```python
from build123d import *

# Parameters (mm, degrees)
F0_W     = 5.588
F0_H     = 23.114
F1_DEPTH = 1.651
F2_W     = 5.75
F2_H     = 23.114
F3_DEPTH = 13.5
F4_R     = 2.1
F5_DEPTH = 25.4
F6_R     = 4
F7_DEPTH = 2.5


with BuildPart() as f1:
    # F0 (on Top) → F1 (new body)
    with BuildSketch(Plane.XY):
        Rectangle(F0_W, F0_H)
    extrude(amount=F1_DEPTH)

    # F2 (on face) → F3 (join)
    with BuildSketch(Plane.XY.offset(1.651)):
        with Locations((3.831, 0)):
            Rectangle(F2_W, F2_H)
    extrude(amount=F3_DEPTH)

    # F4 (on face) → F5 (cut)
    with BuildSketch(Plane.YZ.offset(6.706)):
        with Locations((0, 10.151)):
            Circle(F4_R)
    extrude(amount=-F5_DEPTH, mode=Mode.SUBTRACT)

    # F6 (on face) → F7 (cut)
    with BuildSketch(Plane(origin=(0.956, 0, 0), x_dir=(0, -1, 0), z_dir=(-1, 0, 0))):
        with Locations((0, 10.151)):
            Circle(F6_R)
    extrude(amount=-F7_DEPTH, mode=Mode.SUBTRACT)


solid = f1.part
```
Design review of the part built by this model. Coordinates are the model's own, in mm. A direction names the side the tool comes from. Round coordinates to 2 decimals unless told otherwise and drop trailing zeros. Write each loop counter-clockwise with the first axis right and the second up, starting at its lowest first coordinate (ties: lowest second). Pieces come first, ordered by that corner, then holes. Notation, with made-up numbers: (45.25, -0.75) -> (97.25, -0.75) arc R34 cw to (97.25, 30.25) -> close; hole circle Ø1 at (88.25, 26). An arc over 180 degrees is marked (long way). Answer in a Markdown table with one row per item.
Q1. Take a section at C-C, the plane z = 6.5. State the section outline as (x, y) points, then the cut area to 3 significant figures.
The answers:
| item | result |
|---|---|
| outline | (0.96, -11.56) -> (6.71, -11.56) -> (6.71, 11.56) -> (0.96, 11.56) -> (0.96, 1.63) -> (3.46, 1.63) -> (3.46, -1.63) -> (0.96, -1.63) -> close |
| area | 125 mm² |
Q2. Take a section at B-B, the plane y = -7. State the section outline as (x, z) points, then the cut area to 3 significant figures.
The answers:
| item | result |
|---|---|
| outline | (-2.79, 0) -> (2.79, 0) -> (2.79, 1.65) -> (6.71, 1.65) -> (6.71, 15.15) -> (0.96, 15.15) -> (0.96, 1.65) -> (-2.79, 1.65) -> close |
| area | 86.9 mm² |
Q3. Take a section at D-D, the plane x = 1.75. State the section outline as (y, z) points, then the cut area to 3 significant figures.
The answers:
| item | result |
|---|---|
| outline | (-11.56, 0) -> (11.56, 0) -> (11.56, 15.15) -> (-11.56, 15.15) -> close; hole circle Ø8 at (0, 10.15) |
| area | 300 mm² |
Q4. Take a section at A-A, the plane y = 0. State the section outline as (x, z) points, then the cut area to 3 significant figures.
The answers:
| item | result |
|---|---|
| outline | (-2.79, 0) -> (2.79, 0) -> (2.79, 1.65) -> (6.71, 1.65) -> (6.71, 8.05) -> (3.46, 8.05) -> (3.46, 6.15) -> (0.96, 6.15) -> (0.96, 1.65) -> (-2.79, 1.65) -> close; (0.96, 14.15) -> (3.46, 14.15) -> (3.46, 12.25) -> (6.71, 12.25) -> (6.71, 15.15) -> (0.96, 15.15) -> close |
| area | 53.2 mm² |
Q5. For faces 1 (the face through (2.794, 0, 1)), 2 (the face through (0.956, 0, 5)), 3 (the face through (6.706, 0, 7)), 4 (the face through (3.456, -2, 8)), 5 (the face through (-2.794, 0, 1)), list the 3-axis set-ups (+Z, -Z, +X, -X, +Y, -Y) from which the entire face can be reached by the end or side of a thin tool; tool diameter is ignored.
The answers:
| item | result |
|---|---|
| face 1 | -Z, +X, +Y, -Y |
| face 2 | +Z, -X, +Y, -Y |
| face 3 | +Z, -Z, +X, +Y, -Y |
| face 4 | -X |
| face 5 | +Z, -Z, -X, +Y, -Y |
Q6. To check wall thickness, follow L1, parallel to Z at x = 5.8, y = 0; L2, parallel to Z at x = 1.95, y = 0; L3, parallel to X at y = -4, z = 3. State the ranges of each line that lie inside material, in increasing order. Write a range as [from, to].
The answers:
| item | result |
|---|---|
| L1 | [1.65, 8.05], [12.25, 15.15] |
| L2 | [0, 6.15], [14.15, 15.15] |
| L3 | [0.96, 6.71] |
Q7. Draft analysis for pull direction Z (two halves, no side actions). For faces 6 (the face through (5, 0, 1.651)), 7 (the face through (2.188, 0.521, 14.117)), 8 (the face through (4, -11.557, 7)), state which applies: +Z half, -Z half, draft (parallel to the pull), parting line (faces both ways), or undercut.
The answers:
| item | result |
|---|---|
| face 6 | -Z half |
| face 7 | undercut |
| face 8 | draft |
Q8. Clearance check with flat-ended pins moving along their axes: pin 1 Ø1.2 at (x, y) = (4.5, -2) entering from -Z; pin 2 Ø5 at (y, z) = (0, 10.151) entering from +X; pin 3 Ø1.5 at (x, z) = (0, 13) entering from +Y; pin 4 Ø2.5 at (y, z) = (2, 10.5) entering from -X. State where each tip first meets the part, or that it passes through.
The answers:
| item | result |
|---|---|
| pin 1 | z = 1.65 |
| pin 2 | x = 6.71 |
| pin 3 | through |
| pin 4 | x = 3.46 |
